```python
from build123d import *

# Parameters (mm, degrees)
CROQUIS1_W               = 65
CROQUIS1_H               = 25
SALIENTE_EXTRUIR4_DEPTH  = 13.5
CROQUIS6_W               = 21
CROQUIS6_H               = 11.5
CORTAR_EXTRUIR2_DEPTH    = 65
CROQUIS5_R               = 2
SALIENTE_EXTRUIR6_DEPTH  = 1.5
CROQUIS7_W               = 12
CROQUIS7_H               = 13.5
SALIENTE_EXTRUIR7_DEPTH  = 1.5
CROQUIS8_R               = 5
SALIENTE_EXTRUIR8_DEPTH  = 3
CROQUIS9_R               = 2.5
CORTAR_EXTRUIR3_DEPTH    = 3
CROQUIS10_W              = 6
CROQUIS10_H              = 2
CORTAR_EXTRUIR4_DEPTH    = 10
CROQUIS11_R              = 1.5
CORTAR_EXTRUIR5_DEPTH    = 10
CROQUIS12_R              = 2
CORTAR_EXTRUIR6_DEPTH    = 10
CORTAR_EXTRUIR7_DEPTH    = 2
CROQUIS15_R              = 1.5
CORTAR_EXTRUIR8_DEPTH    = 2
CROQUIS18_R              = 6.5
CORTAR_EXTRUIR9_DEPTH    = 1.8
SALIENTE_EXTRUIR9_DEPTH  = 3
CROQUIS20_W              = 65
CROQUIS20_H              = 1
SALIENTE_EXTRUIR10_DEPTH = 1.5
CROQUIS21_W              = 65
CROQUIS21_H              = 1
SALIENTE_EXTRUIR11_DEPTH = 0.5
CROQUIS22_W              = 65
CROQUIS22_H              = 1
CORTAR_EXTRUIR10_DEPTH   = 0.5


with BuildPart() as part:
    # Croquis1 → Saliente-Extruir4 (new body)
    with BuildSketch(Plane(origin=(0, 0, 0), x_dir=(1, 0, 0), z_dir=(0, 1, 0))):
        with Locations((0, -12.5)):
            Rectangle(CROQUIS1_W, CROQUIS1_H)
    extrude(amount=SALIENTE_EXTRUIR4_DEPTH)

    # Croquis6 → Cortar-Extruir2 (cut)
    with BuildSketch(Plane(origin=(32.5, 0, 0), x_dir=(0, 0, -1), z_dir=(1, 0, 0))):
        with Locations((-12.5, 5.75)):
            Rectangle(CROQUIS6_W, CROQUIS6_H)
    extrude(amount=-CORTAR_EXTRUIR2_DEPTH, mode=Mode.SUBTRACT)

    # Croquis5 → Saliente-Extruir6 (add)
    with BuildSketch(Plane.XY.offset(25)):
        with BuildLine():
            Line((32.5, 0), (32.5, -5.518414164))
            ThreePointArc((32.5, -5.518414164), (32.302775638, -6.384439567), (31.75, -7.079663663))
            ThreePointArc((31.75, -7.079663663), (29.25, -7.957164664), (26.75, -7.079663663))
            ThreePointArc((26.75, -7.079663663), (26.197224362, -6.384439567), (26, -5.518414164))
            Line((26, -5.518414164), (26, 0))
            Line((26, 0), (26, 13.5))
            Line((26, 13.5), (26, 19.018414164))
            ThreePointArc((26, 19.018414164), (26.197224362, 19.884439567), (26.75, 20.579663663))
            ThreePointArc((26.75, 20.579663663), (29.25, 21.457164664), (31.75, 20.579663663))
            ThreePointArc((31.75, 20.579663663), (32.302775638, 19.884439567), (32.5, 19.018414164))
            Line((32.5, 19.018414164), (32.5, 13.5))
            Line((32.5, 13.5), (32.5, 0))
        make_face()
        with Locations((29.25, 17.457164664)):
            Circle(CROQUIS5_R, mode=Mode.SUBTRACT)
        with Locations((29.25, -3.957164664)):
            Circle(CROQUIS5_R, mode=Mode.SUBTRACT)
        with BuildLine():
            Line((-32.5, 0), (-32.5, -5.518414164))
            ThreePointArc((-32.5, -5.518414164), (-32.302775638, -6.384439567), (-31.75, -7.079663663))
            ThreePointArc((-31.75, -7.079663663), (-29.25, -7.957164664), (-26.75, -7.079663663))
            ThreePointArc((-26.75, -7.079663663), (-26.197224362, -6.384439567), (-26, -5.518414164))
            Line((-26, -5.518414164), (-26, 0))
            Line((-26, 0), (-26, 13.5))
            Line((-26, 13.5), (-26, 19.018414164))
            ThreePointArc((-26, 19.018414164), (-26.197224362, 19.884439567), (-26.75, 20.579663663))
            ThreePointArc((-26.75, 20.579663663), (-29.25, 21.457164664), (-31.75, 20.579663663))
            ThreePointArc((-31.75, 20.579663663), (-32.302775638, 19.884439567), (-32.5, 19.018414164))
            Line((-32.5, 19.018414164), (-32.5, 13.5))
            Line((-32.5, 13.5), (-32.5, 0))
        make_face()
    extrude(amount=SALIENTE_EXTRUIR6_DEPTH)

    # Croquis7 → Saliente-Extruir7 (add)
    with BuildSketch(Plane.XY.offset(25)):
        with Locations((0, 6.75)):
            Rectangle(CROQUIS7_W, CROQUIS7_H)
    extrude(amount=SALIENTE_EXTRUIR7_DEPTH)

    # Croquis8 → Saliente-Extruir8 (add)
    with BuildSketch(Plane.XY.offset(26.5)):
        with Locations((0, 6.75)):
            Circle(CROQUIS8_R)
    extrude(amount=SALIENTE_EXTRUIR8_DEPTH)

    # Croquis9 → Cortar-Extruir3 (cut)
    with BuildSketch(Plane.XY.offset(29.5)):
        with Locations((0, 6.75)):
            Circle(CROQUIS9_R)
    extrude(amount=-CORTAR_EXTRUIR3_DEPTH, mode=Mode.SUBTRACT)

    # Croquis10 → Cortar-Extruir4 (cut)
    with BuildSketch(Plane.XZ):
        with Locations((0, 24)):
            Rectangle(CROQUIS10_W, CROQUIS10_H)
    extrude(amount=-CORTAR_EXTRUIR4_DEPTH, mode=Mode.SUBTRACT)

    # Croquis11 → Cortar-Extruir5 (cut)
    with BuildSketch(Plane.XY.offset(26.5)):
        with Locations((0, 6.75)):
            Circle(CROQUIS11_R)
    extrude(amount=-CORTAR_EXTRUIR5_DEPTH, mode=Mode.SUBTRACT)

    # Croquis12 → Cortar-Extruir6 (cut)
    with BuildSketch(Plane.XY.offset(26.5)):
        with Locations((-29.25, 17.5)):
            Circle(CROQUIS12_R)
        with Locations((-29.25, -4)):
            Circle(CROQUIS12_R)
    extrude(amount=-CORTAR_EXTRUIR6_DEPTH, mode=Mode.SUBTRACT)

    # Croquis14 → Cortar-Extruir7 (cut)
    with BuildSketch(Plane(origin=(0, 0, 23), x_dir=(-1, 0, 0), z_dir=(0, 0, -1))):
        with BuildLine():
            Line((-3, 10), (-3, 10.5))
            ThreePointArc((-3, 10.5), (-2.707106781, 11.207106781), (-2, 11.5))
            Line((-2, 11.5), (2, 11.5))
            ThreePointArc((2, 11.5), (2.707106781, 11.207106781), (3, 10.5))
            Line((3, 10.5), (3, 10))
            Line((3, 10), (-3, 10))
        make_face()
    extrude(amount=-CORTAR_EXTRUIR7_DEPTH, mode=Mode.SUBTRACT)

    # Croquis15 → Cortar-Extruir8 (cut)
    with BuildSketch(Plane.XZ.offset(-11.5)):
        with Locations((0, 12.5)):
            Circle(CROQUIS15_R)
    extrude(amount=-CORTAR_EXTRUIR8_DEPTH, mode=Mode.SUBTRACT)

    # Croquis18 → Cortar-Extruir9 (cut)
    with BuildSketch(Plane.XZ.offset(-11.5)):
        with Locations((0, 12.5)):
            Circle(CROQUIS18_R)
    extrude(amount=-CORTAR_EXTRUIR9_DEPTH, mode=Mode.SUBTRACT)

    # Croquis19 → Saliente-Extruir9 (add)
    with BuildSketch(Plane(origin=(0, 13.5, 0), x_dir=(1, 0, 0), z_dir=(0, 1, 0))):
        with BuildLine():
            Line((-3.359531229, -16.203181054), (-4.031437475, -16.943817265))
            ThreePointArc((-4.031437475, -16.943817265), (0, -18.5), (4.031437475, -16.943817265))
            Line((4.031437475, -16.943817265), (3.359531229, -16.203181054))
            ThreePointArc((3.359531229, -16.203181054), (0, -17.5), (-3.359531229, -16.203181054))
        make_face()
        with BuildLine():
            Line((-1.132967397, -6.607938826), (-0.944139498, -7.589949022))
            ThreePointArc((-0.944139498, -7.589949022), (0, -7.5), (0.944139498, -7.589949022))
            Line((0.944139498, -7.589949022), (1.132967397, -6.607938826))
            ThreePointArc((1.132967397, -6.607938826), (0, -6.5), (-1.132967397, -6.607938826))
        make_face()
    extrude(amount=SALIENTE_EXTRUIR9_DEPTH)

    # Croquis20 → Saliente-Extruir10 (add)
    with BuildSketch(Plane.XZ):
        with Locations((0, 0.5)):
            Rectangle(CROQUIS20_W, CROQUIS20_H)
    extrude(amount=SALIENTE_EXTRUIR10_DEPTH)

    # Croquis21 → Saliente-Extruir11 (add)
    with BuildSketch(Plane(origin=(0, 13.5, 0), x_dir=(1, 0, 0), z_dir=(0, 1, 0))):
        with Locations((0, -0.5)):
            Rectangle(CROQUIS21_W, CROQUIS21_H)
    extrude(amount=SALIENTE_EXTRUIR11_DEPTH)

    # Croquis22 → Cortar-Extruir10 (cut)
    with BuildSketch(Plane(origin=(0, 13.5, 0), x_dir=(1, 0, 0), z_dir=(0, 1, 0))):
        with Locations((0, -1.5)):
            Rectangle(CROQUIS22_W, CROQUIS22_H)
    extrude(amount=-CORTAR_EXTRUIR10_DEPTH, mode=Mode.SUBTRACT)


solid = part.part
```
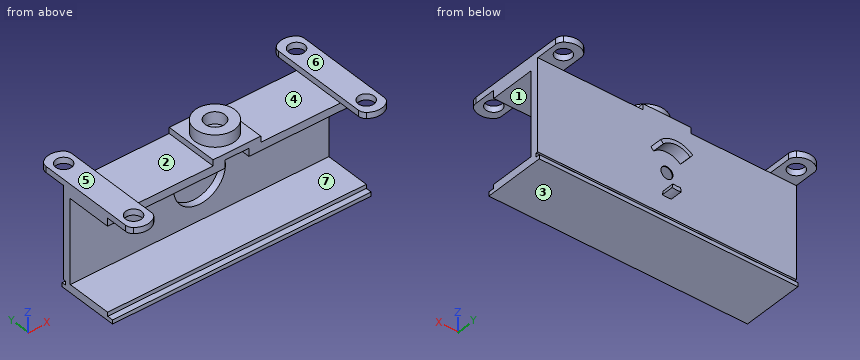
Can you work these out from the model? Positions are in its coordinate system, mm. Face numbers are marked on the shaded views. A direction names the side the tool comes from. Coordinates: 2 decimals unless noted, no trailing zeros. Loops run counter-clockwise (first coordinate to the right, second up) from the corner with the lowest first, then second, coordinate; pieces in that order, holes last. Notation, with made-up numbers: (3.5, 40) - (8.5, 40) arc R20 cw to (8.5, 63) - close; hole circle Ø10 at (10, 60). An arc over 180 degrees is marked (long way). Use a Markdown table: item, result.
Item 1: I want a section at A-A on x = 29.25. Please give me the cut outline in (y, z).
Numbers:
| item | result |
|---|---|
| outline | (-7.96, 25) - (-5.96, 25) - (-5.96, 26.5) - (-7.96, 26.5) - close; (-1.96, 25) - (0, 25) - (0, 23) - (11.5, 23) - (11.5, 2) - (0, 2) - (0, 1) - (-1.5, 1) - (-1.5, 0) - (14, 0) - (14, 1) - (13, 1) - (13, 2) - (13.5, 2) - (13.5, 25) - (15.46, 25) - (15.46, 26.5) - (-1.96, 26.5) - close; (19.46, 25) - (21.46, 25) - (21.46, 26.5) - (19.46, 26.5) - close |
Item 2: For the marked faces 3, 4, 5, 6 and 7, which set-ups out of +Z, -Z, +X, -X, +Y, -Y let a thin tool reach every point of the face, with its end or its side?
Numbers:
| item | result |
|---|---|
| face 3 | -Z, +X, -X, +Y, -Y |
| face 4 | +Z, +Y, -Y |
| face 5 | +Z, -X, +Y, -Y |
| face 6 | +Z, +X, +Y, -Y |
| face 7 | +X, -X, -Y |
Item 3: I want a section at D-D on x = 9. Please give me the cut outline in (y, z), and give its area (3 significant figures).
Numbers:
| item | result |
|---|---|
| outline | (-1.5, 0) - (14, 0) - (14, 1) - (13, 1) - (13, 2) - (13.5, 2) - (13.5, 25) - (0, 25) - (0, 23) - (11.5, 23) - (11.5, 2) - (0, 2) - (0, 1) - (-1.5, 1) - close |
| area | 97.5 mm2 |
Item 4: We'd pull the mould along X, two halves only. Please class the marked faces 1 and 2: released by +X, released by -X, zero draft, split by the parting line, or undercut.
Numbers:
| item | result |
|---|---|
| face 1 | zero draft |
| face 2 | undercut |
Item 5: Will these pins go through, and if not, where does the flat tip stop? pin 1 (5 mm diameter, centred on x = 28.5, y = -5.5, fed in from -Z); pin 2 (0.8 mm diameter, centred on x = -8, z = 0.5, fed in from -Y); pin 3 (11.5 mm diameter, centred on x = 0, z = 12.5, fed in from -Y).
Numbers:
| item | result |
|---|---|
| pin 1 | stops at z = 25 |
| pin 2 | stops at y = -1.5 |
| pin 3 | stops at y = 13.3 |
Item 6: If I drill on probe 1 along Y at (x, z) = (29.25, 25.45); probe 2 along X at (y, z) = (9.5, 25.75); probe 3 along Z at (x, y) = (-20, 2.25), over which ranges is the centre line in solid material (lowest first)? Write a range as from..to.
Numbers:
| item | result |
|---|---|
| probe 1 | y = -7.96..-5.96, -1.96..15.46, 19.46..21.46 |
| probe 2 | x = -32.5..-26, -6..6, 26..32.5 |
| probe 3 | z = 0..2, 23..25 |
Item 7: I want a section at B-B on z = 12.5. Please give me the cut outline in (x, y).
Numbers:
| item | result |
|---|---|
| outline | (-32.5, 11.5) - (-6.5, 11.5) - (-6.5, 13.3) - (-1.5, 13.3) - (-1.5, 13.5) - (-32.5, 13.5) - close; (1.5, 13.3) - (6.5, 13.3) - (6.5, 11.5) - (32.5, 11.5) - (32.5, 13.5) - (1.5, 13.5) - close |
Item 8: I want a section at C-C on y = -4.75. Please give me the cut outline in (x, z), and give its area (3 significant figures).
Numbers:
| item | result |
|---|---|
| outline | (-32.5, 25) - (-31.1, 25) - (-31.1, 26.5) - (-32.5, 26.5) - close; (-27.4, 25) - (-26, 25) - (-26, 26.5) - (-27.4, 26.5) - close; (26, 25) - (27.41, 25) - (27.41, 26.5) - (26, 26.5) - close; (31.09, 25) - (32.5, 25) - (32.5, 26.5) - (31.09, 26.5) - close |
| area | 8.43 mm2 |
